from build123d import *

# Parameters (mm, degrees)
F0_R           = 4.05
F1_DEPTH       = 7
F2_T1_DEPTH    = 63.387088135
F2_T3_DEPTH    = 52.7867319519
F4_DEPTH       = 22
F6_DEPTH       = 5
F7_R           = 4.05
F8_DEPTH       = 2
F9_R           = 4.05
F10_DEPTH      = 3
F11_R          = 4.05
F12_DEPTH      = 5
F13_T4_DEPTH   = 53.0035618315
F14_SIZE       = 2
F17_DEPTH      = 4
F15_R          = 4
F18_DEPTH      = 4.501
F18_DEPTH_BACK = 38.501
F19_R          = 2.3
F20_DEPTH      = 19.5
F21_R          = 2.65
F21_R_2        = 2.3
F22_DEPTH      = 3
F23_R          = 2.15
F24_DEPTH      = 22
F25_R          = 2.65
F25_R_2        = 2.15
F26_DEPTH      = 3
F28_DEPTH      = 1
F30_DEPTH      = 1
F31_R          = 2.1
F32_DEPTH      = 29.501
F33_T1_DEPTH   = 32.387088135
F33_T3_DEPTH   = 13.7849510361
F33_T8_DEPTH   = 29.2867319519
F34_R          = 2.1
F35_DEPTH      = 5


# Not quite as in the source:
# - a fillet or chamfer that OpenCascade refuses, or shapes differently, is made with other operations: its cross-section is extruded or revolved along the edge and cut away or added


with BuildPart() as f1:
    # F0 (on Front) → F1 (new body)
    with BuildSketch(Plane.XZ):
        with BuildLine():
            Line((0, 28.5), (0, 0))
            Line((0, 0), (5, 0))
            Line((5, 0), (5, 21.5))
            Line((5, 21.5), (17, 21.5))
            Line((17, 21.5), (17, -4.5))
            Line((17, -4.5), (59.5, -4.5))
            Line((59.5, -4.5), (59.5, 38.5))
            Line((59.5, 38.5), (10, 38.5))
            ThreePointArc((10, 38.5), (2.9289321881, 35.5710678119), (0, 28.5))
        make_face()
        Polygon((38, -0.5), (38, 9), (55, 9), (55, -0.5), (54.25, -0.5), (54.25, -1.5), (40.25, -1.5), (40.25, -0.5), align=None, mode=Mode.SUBTRACT)
        with Locations((36.95, 17)):
            Circle(F0_R, mode=Mode.SUBTRACT)
        Polygon((28.5, 25), (28.5, 34.5), (30.75, 34.5), (30.75, 35.5), (44.75, 35.5), (44.75, 34.5), (45.5, 34.5), (45.5, 25), align=None, mode=Mode.SUBTRACT)
    extrude(amount=F1_DEPTH)

    # F2: chamfer of 2 on 2 edges, made by hand

    # F2_s2 → F2_t1 (cut)
    with BuildSketch(Plane.YZ.offset(1.2562778409)):
        Polygon((-5, 38.5), (-7, 36.5), (-7, 38.5), align=None)
    extrude(amount=F2_T1_DEPTH, mode=Mode.SUBTRACT)

    # F2_s4 → F2_t3 (cut)
    with BuildSketch(Plane.YZ.offset(11.8566340241)):
        Polygon((-5, -4.5), (-7, -2.5), (-7, -4.5), align=None)
    extrude(amount=F2_T3_DEPTH, mode=Mode.SUBTRACT)

    # F3 (on face) → F4 (join)
    with BuildSketch(Plane(origin=(0, 0, 0), x_dir=(-1, 0, 0), z_dir=(0, 1, 0))):
        with BuildLine():
            Line((-59.5, 21.5), (-17, 21.5))
            Line((-17, 21.5), (-5, 21.5))
            Line((-5, 21.5), (-5, 0))
            Line((-5, 0), (0, 0))
            Line((0, 0), (0, 28.5))
            ThreePointArc((0, 28.5), (-2.9289321881, 35.5710678119), (-10, 38.5))
            Line((-10, 38.5), (-28.5, 38.5))
            Line((-28.5, 38.5), (-28.5, 34.5))
            Line((-28.5, 34.5), (-28.5, 25))
            Line((-28.5, 25), (-45.5, 25))
            Line((-45.5, 25), (-59.5, 25))
            Line((-59.5, 25), (-59.5, 21.5))
        make_face()
    extrude(amount=F4_DEPTH)

    # F5 (on face) → F6 (join)
    with BuildSketch(Plane(origin=(0, 0, 0), x_dir=(-1, 0, 0), z_dir=(0, 1, 0))):
        Polygon((-30.75, 34.5), (-28.5, 34.5), (-28.5, 38.5), (-59.5, 38.5), (-59.5, 34.5), (-45.5, 34.5), (-44.75, 34.5), (-44.75, 35.5), (-30.75, 35.5), align=None)
    extrude(amount=F6_DEPTH)

    # F7 (on face) → F8 (join)
    with BuildSketch(Plane(origin=(0, 0, 0), x_dir=(-1, 0, 0), z_dir=(0, 1, 0))):
        Polygon((-38, 9), (-38, -0.5), (-40.25, -0.5), (-40.25, -1.5), (-54.25, -1.5), (-54.25, -0.5), (-55, -0.5), (-59.5, -0.5), (-59.5, -4.5), (-17, -4.5), (-17, 21.5), (-59.5, 21.5), (-59.5, 9), (-55, 9), align=None)
        with Locations((-36.95, 17)):
            Circle(F7_R, mode=Mode.SUBTRACT)
    extrude(amount=F8_DEPTH)

    # F9 (on face) → F10 (join)
    with BuildSketch(Plane(origin=(0, 2, 0), x_dir=(-1, 0, 0), z_dir=(0, 1, 0))):
        Polygon((-21, -4.5), (-21, 21.5), (-59.5, 21.5), (-59.5, 9), (-38, 9), (-38, -0.5), (-40.25, -0.5), (-40.25, -1.5), (-54.25, -1.5), (-54.25, -0.5), (-59.5, -0.5), (-59.5, -4.5), align=None)
        with Locations((-36.95, 17)):
            Circle(F9_R, mode=Mode.SUBTRACT)
    extrude(amount=F10_DEPTH)

    # F11 (on face) → F12 (join)
    with BuildSketch(Plane(origin=(0, 5, 0), x_dir=(-1, 0, 0), z_dir=(0, 1, 0))):
        Polygon((-38, 9), (-38, -0.5), (-38, -4.5), (-21, -4.5), (-21, 21.5), (-59.5, 21.5), (-59.5, 9), align=None)
        with Locations((-36.95, 17)):
            Circle(F11_R, mode=Mode.SUBTRACT)
    extrude(amount=F12_DEPTH)

    # F13: chamfer of 7 on 1 edges, made by hand


with BuildPart() as f13_tool2:
    # F13_s3 → F13_t4 (new body)
    with BuildSketch(Plane.YZ.offset(56.0017809158)):
        Polygon((3, -4.5), (10, 2.5), (10, -4.5), align=None)
    extrude(amount=-F13_T4_DEPTH)

    split(bisect_by=Plane.YZ.offset(5), keep=Keep.TOP)


with BuildPart() as f1_1:
    add(f1.part)

    # F13_t1: cut F13_tool2
    add(f13_tool2.part, mode=Mode.SUBTRACT)

    # F14
    f14_edges = [f1_1.edges().sort_by_distance(p)[0] for p in [
        (44, 5, 38.5),
        (59.5, 22, 23.25),
    ]]
    chamfer(f14_edges, length=F14_SIZE)

    # F16 (on face) → F17 (cut)
    with BuildSketch(Plane(origin=(21, 0, 0), x_dir=(0, -1, 0), z_dir=(-1, 0, 0))):
        Polygon((-6, 21.5), (-10, 21.5), (-10, 2.5), (-6, -1.5), align=None)
    extrude(amount=-F17_DEPTH, mode=Mode.SUBTRACT)

    # F15 (on Top) → F18 (cut, two sides)
    with BuildSketch(Plane.XY) as f18_sk:
        with Locations((21, 6)):
            Circle(F15_R)
    extrude(amount=-F18_DEPTH, mode=Mode.SUBTRACT)
    extrude(f18_sk.sketch, amount=F18_DEPTH_BACK, mode=Mode.SUBTRACT)

    # F19 (on face) → F20 (cut)
    with BuildSketch(Plane(origin=(0, 0, -4.5), x_dir=(1, 0, 0), z_dir=(0, 0, -1))):
        with Locations((47.25, 0.25)):
            Circle(F19_R)
    extrude(amount=-F20_DEPTH, mode=Mode.SUBTRACT)

    # F21 (on face) → F22 (cut, through all)
    with BuildSketch(Plane(origin=(0, 0, -4.5), x_dir=(1, 0, 0), z_dir=(0, 0, -1))):
        with Locations((47.25, 0.25)):
            Circle(F21_R)
        with Locations((47.25, 0.25)):
            Circle(F21_R_2, mode=Mode.SUBTRACT)
    extrude(amount=-F22_DEPTH, mode=Mode.SUBTRACT)

    # F23 (on face) → F24 (cut)
    with BuildSketch(Plane.XY.offset(38.5)):
        with Locations((37.75, -0.25)):
            Circle(F23_R)
    extrude(amount=-F24_DEPTH, mode=Mode.SUBTRACT)

    # F25 (on face) → F26 (cut, through all)
    with BuildSketch(Plane.XY.offset(38.5)):
        with Locations((37.75, -0.25)):
            Circle(F25_R)
        with Locations((37.75, -0.25)):
            Circle(F25_R_2, mode=Mode.SUBTRACT)
    extrude(amount=-F26_DEPTH, mode=Mode.SUBTRACT)

    # F27 (on face) → F28 (cut)
    with BuildSketch(Plane.XY.offset(25)):
        with BuildLine():
            ThreePointArc((35.8959503782, -7), (32.1832079546, -4.4939163898), (30.75, -0.25))
            Line((30.75, -0.25), (30.75, -7))
            Line((30.75, -7), (35.8959503782, -7))
        make_face()
        with BuildLine():
            ThreePointArc((39.6040496218, -7), (43.3167920454, -4.4939163898), (44.75, -0.25))
            Line((44.75, -0.25), (39.9, -0.25))
            ThreePointArc((39.9, -0.25), (37.75, -2.4), (35.6, -0.25))
            Line((35.6, -0.25), (30.75, -0.25))
            ThreePointArc((30.75, -0.25), (32.1832079546, -4.4939163898), (35.8959503782, -7))
            Line((35.8959503782, -7), (39.6040496218, -7))
        make_face()
        with BuildLine():
            Line((39.9, -0.25), (44.75, -0.25))
            ThreePointArc((44.75, -0.25), (37.75, 6.75), (30.75, -0.25))
            Line((30.75, -0.25), (35.6, -0.25))
            ThreePointArc((35.6, -0.25), (37.75, 1.9), (39.9, -0.25))
        make_face()
        with BuildLine():
            Line((44.75, -7), (44.75, -0.25))
            ThreePointArc((44.75, -0.25), (43.3167920454, -4.4939163898), (39.6040496218, -7))
            Line((39.6040496218, -7), (44.75, -7))
        make_face()
    extrude(amount=-F28_DEPTH, mode=Mode.SUBTRACT)

    # F29 (on face) → F30 (cut)
    with BuildSketch(Plane(origin=(0, 0, 9), x_dir=(1, 0, 0), z_dir=(0, 0, -1))):
        with BuildLine():
            Line((44.95, 0.25), (40.25, 0.25))
            ThreePointArc((40.25, 0.25), (47.25, -6.75), (54.25, 0.25))
            Line((54.25, 0.25), (49.55, 0.25))
            ThreePointArc((49.55, 0.25), (47.25, -2.05), (44.95, 0.25))
        make_face()
        with BuildLine():
            ThreePointArc((45.3959503782, 7), (41.6832079546, 4.4939163898), (40.25, 0.25))
            Line((40.25, 0.25), (44.95, 0.25))
            ThreePointArc((44.95, 0.25), (47.25, 2.55), (49.55, 0.25))
            Line((49.55, 0.25), (54.25, 0.25))
            ThreePointArc((54.25, 0.25), (52.8167920454, 4.4939163898), (49.1040496218, 7))
            Line((49.1040496218, 7), (45.3959503782, 7))
        make_face()
        with BuildLine():
            Line((40.25, 7), (40.25, 0.25))
            ThreePointArc((40.25, 0.25), (41.6832079546, 4.4939163898), (45.3959503782, 7))
            Line((45.3959503782, 7), (40.25, 7))
        make_face()
        with BuildLine():
            ThreePointArc((49.1040496218, 7), (52.8167920454, 4.4939163898), (54.25, 0.25))
            Line((54.25, 0.25), (54.25, 7))
            Line((54.25, 7), (49.1040496218, 7))
        make_face()
    extrude(amount=-F30_DEPTH, mode=Mode.SUBTRACT)

    # F31 (on face) → F32 (cut, through all)
    with BuildSketch(Plane.XY.offset(25)):
        with Locations((36.9, 16)):
            Circle(F31_R)
        with Locations((51.4, 16)):
            Circle(F31_R)
    extrude(amount=-F32_DEPTH, mode=Mode.SUBTRACT)

    # F33: chamfer of 2 on 3 edges, made by hand

    # F33_s2 → F33_t1 (cut)
    with BuildSketch(Plane.YZ.offset(1.2562778409)):
        Polygon((22, 36.5), (20, 38.5), (22, 38.5), align=None)
    extrude(amount=F33_T1_DEPTH, mode=Mode.SUBTRACT)

    # F33_s4 → F33_t3 (cut)
    with BuildSketch(Plane.YZ.offset(50.8584149398)):
        Polygon((5, -2.5), (3, -4.5), (5, -4.5), align=None)
    extrude(amount=F33_T3_DEPTH, mode=Mode.SUBTRACT)


with BuildPart() as f33_tool6:
    # F33_s7 → F33_t8 (new body)
    with BuildSketch(Plane.XZ.offset(-27.1433659759)):
        Polygon((28.5, 36.5), (26.5, 38.5), (28.5, 38.5), align=None)
    extrude(amount=F33_T8_DEPTH)

    split(bisect_by=Plane(origin=(0, 20.75, 20.75), x_dir=(1, 0, 0), z_dir=(0, 0.7071067812, 0.7071067812)), keep=Keep.TOP)


with BuildPart() as f1_2:
    add(f1_1.part)

    # F33_t5: cut F33_tool6
    add(f33_tool6.part, mode=Mode.SUBTRACT)

    # F34 (on face) → F35 (cut, through all)
    with BuildSketch(Plane(origin=(0, 0, 0), x_dir=(0, -1, 0), z_dir=(-1, 0, 0))):
        with Locations((-5, 9.25)):
            Circle(F34_R)
    extrude(amount=-F35_DEPTH, mode=Mode.SUBTRACT)


solid = f1_2.part
Read the model definition and answer for the solid it produces. Units are mm, in the model's axes. A direction names the side the tool comes from. Give positions to 0.01 mm unless a question says otherwise; leave off trailing zeros. Loops run counter-clockwise (first coordinate to the right, second up) from the corner with the lowest first, then second, coordinate; pieces in that order, holes last. Notation, with made-up numbers: (77, 2.5) - (125, 2.5) arc R30 ccw to (125, 39.5) - close; hole circle Ø1 at (-22.75, 14). An arc over 180 degrees is marked (long way). Answer as CSV lines item,"result". Start each with the question number.
1) Determine the mould class of faces 5 (the face through (38, -4, 35.5)), 6 (the face through (31.4, -6, 37.5)), 7 (the face through (37.9, 6.75, 24.51)), 8 (the face through (29, -7, 17)) for opening direction Z: released by +Z, released by -Z, zero draft, split by the parting line, or undercut.
2) Which of the six approach directions +Z, -Z, +X, -X, +Y, -Y give full straight-line access (tool end or side, diameter ignored) to faces 1 (the face through (47.1, 6.75, 9.49)), 2 (the face through (35.103, -0.133, 37.021)), 3 (the face through (45.425, 1.15, 12.465)), 4 (the face through (44, 5, 36))?
3) Straight lines are drawn through the part: L1, parallel to X at y = -4.75, z = 4; L2, parallel to X at y = 8.75, z = 3; L3, parallel to X at y = -5.25, z = 15.5. For each, find the intervals that lie inside material, in ascending order. Write a range as from..to.
4) Find section D-D (x = 36.95). State how many separate pieces and enclosed holes the cut face has, then the cut area to 3 significant figures.
5) Find section B-B (z = 1.5). Write down the section's boundary in (x, y).
6) Find section C-C (y = 13). Write down the section's boundary in (x, z).
7) Each of these flat-tipped pins is pushed along its axis until it touches: pin 1 Ø6 at (x, y) = (34.5, 10.5) entering from -Z; pin 2 Ø4 at (y, z) = (0.5, 33) entering from +X; pin 3 Ø0.5 at (y, z) = (-1.5, -1) entering from -X; pin 4 Ø5 at (x, z) = (36.95, 17) entering from +Y. Where does it stop, or does it pass through?
8) Find section A-A (x = 47.25). Write down the section's boundary in (y, z), then the cut area to 3 significant figures.
Findings below:
1,face 5,"undercut"
1,face 6,"released by +Z"
1,face 7,"undercut"
1,face 8,"zero draft"
2,face 1,"-Y"
2,face 2,"+Z"
2,face 3,"-Z"
2,face 4,"+Z, +X, +Y"
3,L1,"0..5, 17..38, 55..59.5"
3,L2,"0..5, 25..38"
3,L3,"0..5, 17..33.19, 40.71..59.5"
4,separate pieces,"6"
4,enclosed holes,"0"
4,area,"356 mm^2"
5,outline,"(0, -7) - (5, -7) - (5, 22) - (0, 22) - close; (17, -7) - (38, -7) - (38, 9) - (25, 9) - (25, 6) arc R4 cw to (21, 2) - (17, 2) - close; (55, -7) - (59.5, -7) - (59.5, 0) - (55, 0) - close"
6,outline,"(0, 0) - (5, 0) - (5, 21.5) - (59.5, 21.5) - (59.5, 25) - (28.5, 25) - (28.5, 36.5) - (26.5, 38.5) - (10, 38.5) arc R10 ccw to (0, 28.5) - close"
7,pin 1,"z = 0"
7,pin 2,"x = 59.5"
7,pin 3,"x = 17"
7,pin 4,"through"
8,outline,"(-7, -2.5) - (-5, -4.5) - (-2.9, -4.5) - (-2.9, -1.5) - (-7, -1.5) - close; (-7, 10) - (-2.55, 10) - (-2.55, 15) - (2.05, 15) - (2.05, 10) - (6.75, 10) - (6.75, 9) - (10, 9) - (10, 21.5) - (22, 21.5) - (22, 25) - (0, 25) - (0, 34.5) - (5, 34.5) - (5, 36.5) - (3, 38.5) - (-5, 38.5) - (-7, 36.5) - close; (2.4, -4.5) - (3, -4.5) - (5, -2.5) - (5, -1.5) - (2.4, -1.5) - close"
8,area,"404 mm^2"
